from build123d import *

# Parameters (mm, degrees)
SKETCH1_R               = 35
BOSS_EXTRUDE1_DEPTH     = 2
SKETCH3_R               = 6
CUT_EXTRUDE2_DEPTH      = 1
BOSS_EXTRUDE2_DEPTH     = 7.5
CUT_EXTRUDE3_DEPTH      = 50.922439844
CUT_EXTRUDE3_DEPTH_BACK = 50.922439844
SKETCH5_R               = 5
SKETCH6_W               = 23.5
SKETCH6_H               = 26.5
BOSS_EXTRUDE3_DEPTH     = 2.5


with BuildPart() as part:
    # Sketch1 → Boss-Extrude1 (new body)
    with BuildSketch(Plane(origin=(0, 0, 0), x_dir=(1, 0, 0), z_dir=(0, 1, 0))):
        with Locations(Location((0, 0, 0), (0, 0, 270))):
            Circle(SKETCH1_R)
    extrude(amount=BOSS_EXTRUDE1_DEPTH)

    # Sketch3 → Cut-Extrude2 (cut)
    with BuildSketch(Plane(origin=(0, 0, 0), x_dir=(1, 0, 0), z_dir=(0, 1, 0))):
        with Locations(Location((0, 0, 0), (0, 0, 270))):
            Circle(SKETCH3_R)
    extrude(amount=CUT_EXTRUDE2_DEPTH, mode=Mode.SUBTRACT)

    # Sketch4 → Boss-Extrude2 (add)
    with BuildSketch(Plane(origin=(0, 0, 0), x_dir=(1, 0, 0), z_dir=(0, 1, 0))):
        Polygon((-5, 13.5), (-5, 16.5), (-28.5, 16.5), (-28.5, -10), (-5, -10), (-5, -7), (-25.5, -7), (-25.5, 13.5), align=None)
    extrude(amount=BOSS_EXTRUDE2_DEPTH)

    # Sketch5 → Cut-Extrude3 (cut, two sides: drawn at the far end of the back side and taken through both)
    with BuildSketch(Plane.XZ.offset(-1).offset(-CUT_EXTRUDE3_DEPTH_BACK)):
        with Locations(Location((0, 0, 0), (0, 0, 270))):
            Circle(SKETCH5_R)
    extrude(amount=CUT_EXTRUDE3_DEPTH + CUT_EXTRUDE3_DEPTH_BACK, mode=Mode.SUBTRACT)

    # Sketch6 → Boss-Extrude3 (add)
    with BuildSketch(Plane(origin=(0, 2, 0), x_dir=(1, 0, 0), z_dir=(0, 1, 0))):
        with Locations((-16.75, 3.25)):
            Rectangle(SKETCH6_W, SKETCH6_H)
    extrude(amount=BOSS_EXTRUDE3_DEPTH)


solid = part.part
Read the model definition and answer for the solid it produces. Units are mm, in the model's axes. A direction names the side the tool comes from. Coordinates: 2 decimals unless noted, no trailing zeros. Loops run counter-clockwise (first coordinate to the right, second up) from the corner with the lowest first, then second, coordinate; pieces in that order, holes last. Notation, with made-up numbers: (31, 40) -> (59, 40) arc R8 cw to (59, 51) -> close; hole circle Ø6 at (-31.5, -6). An arc over 180 degrees is marked (long way). Answer in a Markdown table with one row per item.
Item 1: A cutting plane is placed at C-C on x = -21. Determine the outline of the cut face in (y, z).
Returned:
| item | result |
|---|---|
| outline | (0, -28) -> (2, -28) -> (2, -16.5) -> (7.5, -16.5) -> (7.5, -13.5) -> (4.5, -13.5) -> (4.5, 7) -> (7.5, 7) -> (7.5, 10) -> (2, 10) -> (2, 28) -> (0, 28) -> close |
Item 2: Straight lines are drawn through the part: line 1 along X through (y, z) = (1.3, 0); line 2 along Z through (x, y) = (-22, 6.75); line 3 along X through (y, z) = (0.85, 0). For each, find the intervals that lie inside material, in ascending order. Write a range as [from, to].
Returned:
| item | result |
|---|---|
| line 1 | x = [-35, -5], [5, 35] |
| line 2 | z = [-16.5, -13.5], [7, 10] |
| line 3 | x = [-35, -6], [6, 35] |
Item 3: A cutting plane is placed at A-A on x = 0. Determine the outline of the cut face in (y, z), plus the area to 3 significant figures.
Returned:
| item | result |
|---|---|
| outline | (0, -35) -> (2, -35) -> (2, -5) -> (1, -5) -> (1, -6) -> (0, -6) -> close; (0, 6) -> (1, 6) -> (1, 5) -> (2, 5) -> (2, 35) -> (0, 35) -> close |
| area | 118 mm^2 |
Item 4: A cutting plane is placed at B-B on z = 1. Determine the outline of the cut face in (x, y), plus the area to 3 significant figures.
Returned:
| item | result |
|---|---|
| outline | (-34.99, 0) -> (-5.92, 0) -> (-5.92, 1) -> (-4.9, 1) -> (-4.9, 2) -> (-5, 2) -> (-5, 4.5) -> (-25.5, 4.5) -> (-25.5, 7.5) -> (-28.5, 7.5) -> (-28.5, 2) -> (-34.99, 2) -> close; (4.9, 1) -> (5.92, 1) -> (5.92, 0) -> (34.99, 0) -> (34.99, 2) -> (4.9, 2) -> close |
| area | 186 mm^2 |
Item 5: Each of these flat-tipped pins is pushed along its axis until it touches: P1, Ø4.5, axis at y = 3.5, z = -7, coming from the +X side; P2, Ø16, axis at x = 0, z = 0, coming from the +Y side; P3, Ø5, axis at x = 15.5, z = -17, coming from the +Y side. Where does it stop, or does it pass through?
Returned:
| item | result |
|---|---|
| P1 | stops at x = 34.59 |
| P2 | stops at y = 4.5 |
| P3 | stops at y = 2 |
Item 6: For faces 1 (the flat face through (-17, 5, -16.5)), 2 (the flat face through (-15, 6, 7)), 3 (the flat face through (4, 1, -4)), 4 (the flat face through (-5, 3, -3)), determine the directions among +Z, -Z, +X, -X, +Y, -Y from which every point of the face is accessible in a straight line to the end or side of a thin tool.
Returned:
| item | result |
|---|---|
| face 1 | -Z, +X, -X, +Y |
| face 2 | +X, +Y |
| face 3 | -Y |
| face 4 | +Z, -Z, +X, +Y |
Item 7: A cutting plane is placed at D-D on z = -12. Determine the outline of the cut face in (x, y), plus the area to 3 significant figures.
Returned:
| item | result |
|---|---|
| outline | (-32.88, 0) -> (32.88, 0) -> (32.88, 2) -> (-5, 2) -> (-5, 4.5) -> (-25.5, 4.5) -> (-25.5, 7.5) -> (-28.5, 7.5) -> (-28.5, 2) -> (-32.88, 2) -> close |
| area | 199 mm^2 |
Item 8: For a pull along X with two mould halves and no side action, classify faces 5 (the flat face through (-17, 5, 10)), 6 (the cylindrical face through (1.802, 0.493, 5.723)), 7 (the flat face through (-28.5, 5, -3)) as released by +X, released by -X, zero draft, split by the parting line, or undercut.
Returned:
| item | result |
|---|---|
| face 5 | zero draft |
| face 6 | undercut |
| face 7 | released by -X |
